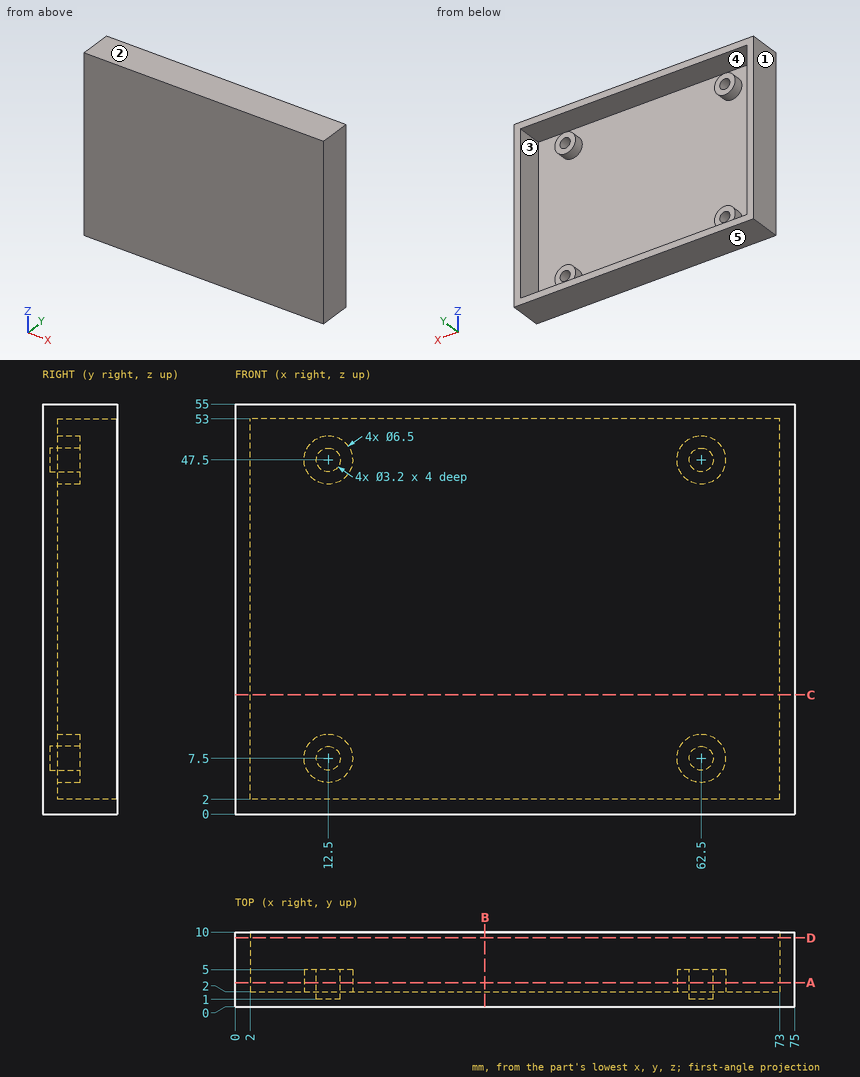
Print and shaded views of the part. All mm, measured from the part's lowest x, y and z. A direction names the side the tool comes from. Give positions to 0.01 mm unless a question says otherwise; leave off trailing zeros. Loops run counter-clockwise (first coordinate to the right, second up) from the corner with the lowest first, then second, coordinate; pieces in that order, holes last.
1) Tool access for the marked faces 4 and 5: list every direction of +Z, -Z, +X, -X, +Y, -Y with a clear straight run to the whole face (end or side of a thin tool).
2) Flat gauge pins, fed straight in: pin 1 Ø1.6 at (x, z) = (13, 48) entering from +Y; pin 2 Ø4 at (x, z) = (31.5, 35.5) entering from +Y; pin 3 Ø4 at (x, z) = (62.5, 47.5) entering from +Y. Where does each tip first touch, or does it go through?
3) Saw through at A-A (y = 3.25). Count the separate pieces of the cut face and the enclosed holes in it, plus the area to 3 significant figures.
4) Pull direction Z, two halves, no side cores. Call the marked faces 1, 2 and 3: +Z half, -Z half, draft (parallel to the pull), parting line (faces both ways), or undercut.
5) Saw through at C-C (z = 16). Write the cut outline in (x, y), plus the area to 3 significant figures.
6) Saw through at B-B (x = 33.5). Write the cut outline in (y, z).
7) Wall check: line 1 (X direction, y = 4.05, z = 7.5); line 2 (X direction, y = 9.75, z = 23); line 3 (Z direction, x = 64, y = 9.75). Give the ranges that are in metal, low to high.
8) Saw through at D-D (y = 9.25). Write the cut outline in (x, z), plus the area to 3 significant figures.
Answer block:
1. face 4: +Y
1. face 5: -Z, +X, -X, +Y, -Y
2. pin 1: stops at y = 1
2. pin 2: stops at y = 2
2. pin 3: stops at y = 5
3. separate pieces: 5
3. enclosed holes: 5
3. area: 605 mm2
4. face 1: draft
4. face 2: +Z half
4. face 3: undercut
5. outline: (0, 0) - (75, 0) - (75, 10) - (73, 10) - (73, 2) - (2, 2) - (2, 10) - (0, 10) - close
5. area: 182 mm2
6. outline: (0, 0) - (10, 0) - (10, 2) - (2, 2) - (2, 53) - (10, 53) - (10, 55) - (0, 55) - close
7. line 1: x = 0 to 2, 9.25 to 10.9, 14.1 to 15.75, 59.25 to 60.9, 64.1 to 65.75, 73 to 75
7. line 2: x = 0 to 2, 73 to 75
7. line 3: z = 0 to 2, 53 to 55
8. outline: (0, 0) - (75, 0) - (75, 55) - (0, 55) - close; hole (2, 2) - (73, 2) - (73, 53) - (2, 53) - close
8. area: 504 mm2
